```python
from build123d import *

# Parameters (mm, degrees)
ESQUISSE1_R      = 5.25
ESQUISSE1_R_2    = 2.25
ESQUISSE1_R_3    = 2.5
EXTRUSION1_DEPTH = 3


with BuildPart() as part:
    # Esquisse1 → Extrusion1 (new body)
    with BuildSketch(Plane(origin=(0, 0, 0), x_dir=(1, 0, 0), z_dir=(0, 1, 0))):
        with BuildLine():
            Line((-64.494367887, 52.858171056), (-99, 26))
            Line((-99, 26), (-106, 26))
            Line((-106, 26), (-106, 39))
            Line((-106, 39), (-125, 39))
            Line((-125, 39), (-125, 26))
            Line((-125, 26), (-132, 26))
            Line((-132, 26), (-132, 95))
            Line((-132, 95), (-87, 95))
            Line((-87, 95), (-77, 85))
            Line((-77, 85), (-67, 85))
            Line((-67, 85), (-57, 95))
            Line((-57, 95), (57, 95))
            Line((57, 95), (67, 85))
            Line((67, 85), (77, 85))
            Line((77, 85), (87, 95))
            Line((87, 95), (132, 95))
            Line((132, 95), (132, 26))
            Line((132, 26), (125, 26))
            Line((125, 26), (125, 39))
            Line((125, 39), (106, 39))
            Line((106, 39), (106, 26))
            Line((106, 26), (99, 26))
            Line((99, 26), (64.494367887, 52.858171056))
            ThreePointArc((64.494367887, 52.858171056), (0, 75), (-64.494367887, 52.858171056))
        make_face()
        with Locations((-117, 80)):
            Circle(ESQUISSE1_R, mode=Mode.SUBTRACT)
        with Locations((117, 80)):
            Circle(ESQUISSE1_R, mode=Mode.SUBTRACT)
        with Locations((-127.253048327, 90.253048327)):
            Circle(ESQUISSE1_R_2, mode=Mode.SUBTRACT)
        with Locations((-106.746951673, 90.253048327)):
            Circle(ESQUISSE1_R_2, mode=Mode.SUBTRACT)
        with Locations((-106.746951673, 69.746951673)):
            Circle(ESQUISSE1_R_2, mode=Mode.SUBTRACT)
        with Locations((-127.253048327, 69.746951673)):
            Circle(ESQUISSE1_R_2, mode=Mode.SUBTRACT)
        with Locations((106.746951673, 69.746951673)):
            Circle(ESQUISSE1_R_2, mode=Mode.SUBTRACT)
        with Locations((127.253048327, 69.746951673)):
            Circle(ESQUISSE1_R_2, mode=Mode.SUBTRACT)
        with Locations((127.253048327, 90.253048327)):
            Circle(ESQUISSE1_R_2, mode=Mode.SUBTRACT)
        with Locations((106.746951673, 90.253048327)):
            Circle(ESQUISSE1_R_2, mode=Mode.SUBTRACT)
        with Locations((-70.636688638, 60.749425443)):
            Circle(ESQUISSE1_R_3, mode=Mode.SUBTRACT)
        with Locations((70.636688638, 60.749425443)):
            Circle(ESQUISSE1_R_3, mode=Mode.SUBTRACT)
        with Locations((0, 85)):
            Circle(ESQUISSE1_R_3, mode=Mode.SUBTRACT)
    extrude(amount=EXTRUSION1_DEPTH)


solid = part.part
```
Source: CAD feature listing. Evaluate the final solid. Frame: model axes, mm. A direction names the side the tool comes from. Coordinates: 2 decimals unless noted, no trailing zeros. Loops run counter-clockwise (first coordinate to the right, second up) from the corner with the lowest first, then second, coordinate; pieces in that order, holes last. Notation, with made-up numbers: M 37.5,53.5 L 46.5,53.5 A27 cw 46.5,73.5 Z; hole C 86,42 d2. An arc over 180 degrees is marked long. Put each result on its own line as item: value. Start each with the question number.
1) Reachability of faces 5 (the face through (-72.48, 1.48, -62.44)), 6 (the face through (-82, 1, -90)), 7 (the face through (81.99, 1.48, -39.24)) from +Z, -Z, +X, -X, +Y, -Y: full face, straight path, thin tool, end or side. Return the list, or none.
2) Cut plane A-A on x = -117. Return the cut outline in (y, z), then the cut area to 4 significant figures.
3) Contact query for flat-ended pins moving along their axis: pin 1 Ø7 at (x, z) = (-127.25, -69.75) entering from +Y; pin 2 Ø1 at (x, y) = (53.5, 1.5) entering from +Z; pin 3 Ø1.5 at (x, y) = (-85, 2.5) entering from +Z; pin 4 Ø1.5 at (x, y) = (-74, 1) entering from -Z. Output: stop coordinate, or through.
4) Cut plane B-B on z = -80. Return the cut outline in (x, y), then the cut area to 3 significant figures.
5) Cut plane D-D on x = 0. Return the cut outline in (y, z), then the cut area to 3 significant figures.
6) Ray query, L1, parallel to X at y = 2.55, z = -34; L2, parallel to X at y = 0.5, z = -86; L3, parallel to X at y = 1.7, z = -50. Return the intervals inside material, ascending. Write a range as from..to.
7) Pull-direction query (Z, two-part tool) for faces 1 (the face through (2, 3, -76)), 2 (the face through (-112, 1.5, -81.6)), 3 (the face through (-62, 1, -90)), 4 (the face through (-81.506, 1.479, -39.617)); classes: pulls with the +Z half, pulls with the -Z half, needs draft (parallel to the pull), parting line crosses it, or undercut.
8) Cut plane C-C on z = -34. Return the cut outline in (x, y).
The answers:
1. face 5: +Y, -Y
1. face 6: -Z, +Y, -Y
1. face 7: +Z, +Y, -Y
2. outline: M 0,-95 L 3,-95 L 3,-85.25 L 0,-85.25 Z; M 0,-74.75 L 3,-74.75 L 3,-39 L 0,-39 Z
2. area: 136.5 mm²
3. pin 1: stops at y = 3
3. pin 2: stops at z = -60.05
3. pin 3: stops at z = -36.31
3. pin 4: stops at z = -85
4. outline: M -132,0 L -122.25,0 L -122.25,3 L -132,3 Z; M -111.75,0 L 111.75,0 L 111.75,3 L -111.75,3 Z; M 122.25,0 L 132,0 L 132,3 L 122.25,3 Z
4. area: 729 mm²
5. outline: M 0,-95 L 3,-95 L 3,-87.5 L 0,-87.5 Z; M 0,-82.5 L 3,-82.5 L 3,-75 L 0,-75 Z
5. area: 45.0 mm²
6. L1: x = -132..-125, -106..-88.72, 88.72..106, 125..132
6. L2: x = -132..-78, -66..-2.29, 2.29..66, 78..132
6. L3: x = -132..-68.17, 68.17..132
7. face 1: needs draft
7. face 2: undercut
7. face 3: pulls with the -Z half
7. face 4: pulls with the +Z half
8. outline: M -132,0 L -125,0 L -125,3 L -132,3 Z; M -106,0 L -88.72,0 L -88.72,3 L -106,3 Z; M 88.72,0 L 106,0 L 106,3 L 88.72,3 Z; M 125,0 L 132,0 L 132,3 L 125,3 Z
